```python
from build123d import *

# Parameters (mm, degrees)
SKETCH_1_W          = 15
SKETCH_1_H          = 180
SKETCH_1_R          = 2
EXTRUDE_1_DEPTH     = 15
SKETCH_2_R          = 3.75
CUT_EXTRUDE_1_DEPTH = 5


with BuildPart() as part:
    # Эскиз1 → Бобышка-Вытянуть1 (new body)
    with BuildSketch(Plane(origin=(0, 0, 0), x_dir=(1, 0, 0), z_dir=(0, 1, 0))):
        with Locations((-55.055059152, 159.322347884)):
            Rectangle(SKETCH_1_W, SKETCH_1_H)
        with Locations(Location((-55.055059152, 219.219125448, 0), (0, 0, 270))):
            Circle(SKETCH_1_R, mode=Mode.SUBTRACT)
        with Locations(Location((-55.055059152, 159.219125448, 0), (0, 0, 270))):
            Circle(SKETCH_1_R, mode=Mode.SUBTRACT)
        with Locations(Location((-55.055059152, 99.219125448, 0), (0, 0, 270))):
            Circle(SKETCH_1_R, mode=Mode.SUBTRACT)
    extrude(amount=EXTRUDE_1_DEPTH)

    # Эскиз2 → Вырез-Вытянуть1 (cut)
    with BuildSketch(Plane(origin=(0, 15, 0), x_dir=(1, 0, 0), z_dir=(0, 1, 0))):
        with Locations(Location((-55.055059152, 99.219125448, 0), (0, 0, 270))):
            Circle(SKETCH_2_R)
        with Locations(Location((-55.055059152, 159.219125448, 0), (0, 0, 270))):
            Circle(SKETCH_2_R)
        with Locations(Location((-55.055059152, 219.219125448, 0), (0, 0, 270))):
            Circle(SKETCH_2_R)
    extrude(amount=-CUT_EXTRUDE_1_DEPTH, mode=Mode.SUBTRACT)


solid = part.part
```
Can you work these out from the model? Positions are in its coordinate system, mm. A direction names the side the tool comes from. Coordinates: 2 decimals unless noted, no trailing zeros. Put each result on its own line as item: value. Start each with the question number.
(1) We'd pull the mould along X, two halves only. Please class faces 3 (the face through (-62.555, 7, -158)), 4 (the face through (-57.337, 12.535, -222.195)), 5 (the face through (-47.555, 7, -158)), 6 (the face through (-55, 7, -69.322)): +X half, -X half, draft (parallel to the pull), parting line (faces both ways), or undercut.
(2) Will these pins go through, and if not, where does the flat tip stop? pin 1 Ø4 at (x, z) = (-56, -218) entering from +Y; pin 2 Ø2.5 at (x, z) = (-55.06, -219.22) entering from +Y.
(3) I need wall thicknesses on probe 1 along Z at (x, y) = (-55.75, 10.25); probe 2 along Z at (x, y) = (-54, 5.5). Which ranges of each line are inside material? Lowest first, please.
(4) Which directions (+Z, -Z, +X, -X, +Y, -Y) give clear straight access to the entire face, cutting with the end or side of a thin tool? Please do faces 1 (the face through (-57, 10, -158)), 2 (the face through (-56.27, 4.93, -100.81)).
Worked answers:
1. face 3: -X half
1. face 4: undercut
1. face 5: +X half
1. face 6: draft
2. pin 1: stops at y = 10
2. pin 2: passes through
3. probe 1: z = -249.32 to -222.9, -215.53 to -162.9, -155.53 to -102.9, -95.53 to -69.32
3. probe 2: z = -249.32 to -220.92, -217.52 to -160.92, -157.52 to -100.92, -97.52 to -69.32
4. face 1: +Y
4. face 2: +Y, -Y
